The listing builds one solid part. Answer for the finished solid, in the listing's coordinates (mm). A direction names the side the tool comes from. Give positions to 0.01 mm unless a question says otherwise; leave off trailing zeros. Order: outer loops, then holes, each group sorted by start corner. A loop starts at its lowest first (then second) coordinate and runs counter-clockwise, first axis right, second up.
```python
from build123d import *

# Parameters (mm, degrees)
ESQUISSE1_W              = 150
ESQUISSE1_H              = 240
BOSS_EXTRU_1_DEPTH       = 50
ENL_V_MAT_EXTRU_1_DEPTH  = 42
ESQUISSE3_W              = 101
ESQUISSE3_H              = 165.5
ENL_V_MAT_EXTRU_2_DEPTH  = 151.083310198
CONG_1_R                 = 5
ESQUISSE4_R              = 2.8
ENL_V_MAT_EXTRU_3_DEPTH  = 15
ENL_V_MAT_EXTRU_4_DEPTH  = 199.494332413
ESQUISSE7_R              = 2.3
ENL_V_MAT_EXTRU_5_DEPTH  = 5
ESQUISSE6_R              = 2
ENL_V_MAT_EXTRU_6_DEPTH  = 5
ESQUISSE8_W              = 5
ESQUISSE8_H              = 40
ENL_V_MAT_EXTRU_7_DEPTH  = 7
ESQUISSE9_R              = 4
BOSS_EXTRU_2_DEPTH       = 9
ESQUISSE10_R             = 2.3
ENL_V_MAT_EXTRU_8_DEPTH  = 8
ESQUISSE11_W             = 101
ESQUISSE11_H             = 11
ENL_V_MAT_EXTRU_9_DEPTH  = 3
BOSS_EXTRU_3_START       = 10
ESQUISSE13_R             = 4
ESQUISSE13_R_2           = 2.3
ESQUISSE13_R_3           = 2
BOSS_EXTRU_3_DEPTH       = 10
ESQUISSE14_R             = 2.3
ENL_V_MAT_EXTRU_10_DEPTH = 6.7


with BuildPart() as part:
    # Esquisse1 → Boss.-Extru.1 (new body)
    with BuildSketch(Plane.XY):
        Rectangle(ESQUISSE1_W, ESQUISSE1_H)
    extrude(amount=BOSS_EXTRU_1_DEPTH)

    # Esquisse2 → Enl_v. mat.-Extru.1 (cut)
    with BuildSketch(Plane(origin=(0, 0, 0), x_dir=(-1, 0, 0), z_dir=(0, 0, -1))):
        with BuildLine():
            Line((-70, -110), (-70, 110))
            Line((-70, 110), (-67, 110))
            ThreePointArc((-67, 110), (-65.585786438, 110.585786438), (-65, 112))
            Line((-65, 112), (-65, 115))
            Line((-65, 115), (65, 115))
            Line((65, 115), (65, 112))
            ThreePointArc((65, 112), (65.585786438, 110.585786438), (67, 110))
            Line((67, 110), (70, 110))
            Line((70, 110), (70, -110))
            Line((70, -110), (26, -110))
            ThreePointArc((26, -110), (25.292893219, -110.292893219), (25, -111))
            Line((25, -111), (25, -115))
            Line((25, -115), (-65, -115))
            Line((-65, -115), (-65, -112))
            ThreePointArc((-65, -112), (-65.585786438, -110.585786438), (-67, -110))
            Line((-67, -110), (-70, -110))
        make_face()
    extrude(amount=-ENL_V_MAT_EXTRU_1_DEPTH, mode=Mode.SUBTRACT)

    # Esquisse3 → Enl_v. mat.-Extru.2 (cut, through all)
    with BuildSketch(Plane.XY.offset(50)):
        with Locations((0, 27.25)):
            Rectangle(ESQUISSE3_W, ESQUISSE3_H)
    extrude(amount=-ENL_V_MAT_EXTRU_2_DEPTH, mode=Mode.SUBTRACT)

    # Cong_1
    cong_1_edges = [part.edges().sort_by_distance(p)[0] for p in [
        (-75, 120, 25),
        (75, 120, 25),
        (75, -120, 25),
        (-75, -120, 25),
    ]]
    fillet(cong_1_edges, radius=CONG_1_R)

    # Esquisse4 → Enl_v. mat.-Extru.3 (cut)
    with BuildSketch(Plane(origin=(0, 0, 0), x_dir=(-1, 0, 0), z_dir=(0, 0, -1))):
        with Locations((-70, 115)):
            Circle(ESQUISSE4_R)
        with Locations((70, 115)):
            Circle(ESQUISSE4_R)
        with Locations((70, -115)):
            Circle(ESQUISSE4_R)
        with Locations((-70, -115)):
            Circle(ESQUISSE4_R)
    extrude(amount=-ENL_V_MAT_EXTRU_3_DEPTH, mode=Mode.SUBTRACT)

    # Esquisse5 → Enl_v. mat.-Extru.4 (cut, through all)
    with BuildSketch(Plane(origin=(75, 0, 0), x_dir=(0, 0, -1), z_dir=(1, 0, 0))):
        with BuildLine():
            Line((-37, 55), (-18.584929033, 78.683014193))
            ThreePointArc((-18.584929033, 78.683014193), (-14.375120517, 79.209808516), (-13.848326194, 75))
            Line((-13.848326194, 75), (-32.263397161, 51.316985807))
            ThreePointArc((-32.263397161, 51.316985807), (-36.473205677, 50.790191484), (-37, 55))
        make_face()
        with BuildLine():
            Line((-37, 5), (-18.584929033, 28.683014193))
            ThreePointArc((-18.584929033, 28.683014193), (-14.375120517, 29.209808516), (-13.848326194, 25))
            Line((-13.848326194, 25), (-32.263397161, 1.316985807))
            ThreePointArc((-32.263397161, 1.316985807), (-36.473205677, 0.790191484), (-37, 5))
        make_face()
        with BuildLine():
            Line((-37, -45), (-18.584929033, -21.316985807))
            ThreePointArc((-18.584929033, -21.316985807), (-14.375120517, -20.790191484), (-13.848326194, -25))
            Line((-13.848326194, -25), (-32.263397161, -48.683014193))
            ThreePointArc((-32.263397161, -48.683014193), (-36.473205677, -49.209808516), (-37, -45))
        make_face()
    extrude(amount=-ENL_V_MAT_EXTRU_4_DEPTH, mode=Mode.SUBTRACT)

    # Esquisse7 → Enl_v. mat.-Extru.5 (cut)
    with BuildSketch(Plane(origin=(0, 0, 42), x_dir=(-1, 0, 0), z_dir=(0, 0, -1))):
        with Locations((-57, 105.8)):
            Circle(ESQUISSE7_R)
        with Locations((-57, -51.3)):
            Circle(ESQUISSE7_R)
        with Locations((57, 105.8)):
            Circle(ESQUISSE7_R)
        with Locations((57, -51.3)):
            Circle(ESQUISSE7_R)
    extrude(amount=-ENL_V_MAT_EXTRU_5_DEPTH, mode=Mode.SUBTRACT)

    # Esquisse6 → Enl_v. mat.-Extru.6 (cut)
    with BuildSketch(Plane(origin=(0, 0, 42), x_dir=(-1, 0, 0), z_dir=(0, 0, -1))):
        with Locations((-14.8, -79.815913119)):
            Circle(ESQUISSE6_R)
        with Locations((13, -105.015913119)):
            Circle(ESQUISSE6_R)
    extrude(amount=-ENL_V_MAT_EXTRU_6_DEPTH, mode=Mode.SUBTRACT)

    # Esquisse8 → Enl_v. mat.-Extru.7 (cut)
    with BuildSketch(Plane(origin=(0, 0, 42), x_dir=(-1, 0, 0), z_dir=(0, 0, -1))):
        with Locations((53, -27.5)):
            Rectangle(ESQUISSE8_W, ESQUISSE8_H)
    extrude(amount=-ENL_V_MAT_EXTRU_7_DEPTH, mode=Mode.SUBTRACT)

    # Esquisse9 → Boss.-Extru.2 (add)
    with BuildSketch(Plane(origin=(0, 0, 42), x_dir=(-1, 0, 0), z_dir=(0, 0, -1))):
        with Locations((-60, 97)):
            Circle(ESQUISSE9_R)
        with Locations((60, 97)):
            Circle(ESQUISSE9_R)
        with Locations((60, -33)):
            Circle(ESQUISSE9_R)
        with Locations((-60, -33)):
            Circle(ESQUISSE9_R)
    extrude(amount=BOSS_EXTRU_2_DEPTH)

    # Esquisse10 → Enl_v. mat.-Extru.8 (cut)
    with BuildSketch(Plane(origin=(0, 0, 33), x_dir=(-1, 0, 0), z_dir=(0, 0, -1))):
        with Locations((-60, 97)):
            Circle(ESQUISSE10_R)
        with Locations((60, 97)):
            Circle(ESQUISSE10_R)
        with Locations((60, -33)):
            Circle(ESQUISSE10_R)
        with Locations((-60, -33)):
            Circle(ESQUISSE10_R)
    extrude(amount=-ENL_V_MAT_EXTRU_8_DEPTH, mode=Mode.SUBTRACT)

    # Esquisse11 → Enl_v. mat.-Extru.9 (cut)
    with BuildSketch(Plane(origin=(0, 0, 42), x_dir=(-1, 0, 0), z_dir=(0, 0, -1))):
        with Locations((0, -61)):
            Rectangle(ESQUISSE11_W, ESQUISSE11_H)
    extrude(amount=-ENL_V_MAT_EXTRU_9_DEPTH, mode=Mode.SUBTRACT)

    # Esquisse13 → Boss.-Extru.3 (add)
    # profile 1 of 2: a face of its own
    with BuildSketch(Plane(origin=(0, 0, 42), x_dir=(-1, 0, 0), z_dir=(0, 0, -1)).offset(BOSS_EXTRU_3_START)):
        with Locations((-14.8, -79.815913119)):
            Circle(ESQUISSE13_R)
        with Locations((-14.8, -79.815913119)):
            Circle(ESQUISSE13_R_2, mode=Mode.SUBTRACT)
    # profile 2 of 2: a face of its own
    with BuildSketch(Plane(origin=(0, 0, 42), x_dir=(-1, 0, 0), z_dir=(0, 0, -1)).offset(BOSS_EXTRU_3_START)):
        with Locations((13, -105.015913119)):
            Circle(ESQUISSE13_R)
        with Locations((13, -105.015913119)):
            Circle(ESQUISSE13_R_3, mode=Mode.SUBTRACT)
    extrude(amount=-BOSS_EXTRU_3_DEPTH)

    # Esquisse14 → Enl_v. mat.-Extru.10 (cut)
    with BuildSketch(Plane(origin=(0, -110, 0), x_dir=(1, 0, 0), z_dir=(0, 1, 0))):
        with Locations(Location((-63.627600244, -37.7, 0), (0, 0, 180))):
            Circle(ESQUISSE14_R)
        with Locations(Location((-63.627600244, -4.8, 0), (0, 0, 180))):
            Circle(ESQUISSE14_R)
        with Locations(Location((-20.327600244, -4.8, 0), (0, 0, 180))):
            Circle(ESQUISSE14_R)
    extrude(amount=-ENL_V_MAT_EXTRU_10_DEPTH, mode=Mode.SUBTRACT)


solid = part.part
```
1) Straight lines are drawn through the part: probe 1 along Y at (x, z) = (57, 45.3); probe 2 along Y at (x, z) = (-17, 30.5); probe 3 along Y at (x, z) = (56.5, 46.5) (3 decimals). For each, find the intervals that lie inside material, in ascending order.
Geometry says:
probe 1: y = -120 to -53.6, -49 to 103.5, 108.1 to 120
probe 2: y = -120 to -115, 115 to 120
probe 3: y = -120 to -53.545, -49.055 to 103.555, 108.045 to 120
2) Find section A-A (y = 46). Write down the section's boundary in (x, z), then the cut area to 3 significant figures.
Geometry says:
outline: (-75, 0) - (-70, 0) - (-70, 42) - (-50.5, 42) - (-50.5, 50) - (-75, 50) - close; (50.5, 42) - (70, 42) - (70, 0) - (75, 0) - (75, 50) - (50.5, 50) - close
area: 812 mm2
3) For a pull along Y with two mould halves and no side action, classify faces 4 (the cylindrical face through (-74, 118, 25)), 5 (the flat face through (72.5, -33.3, 27.9)) as +Y half, -Y half, draft (parallel to the pull), parting line (faces both ways), or undercut.
Geometry says:
face 4: +Y half
face 5: undercut
4) Find section B-B (x = -40). Write down the section's boundary in (y, z), then the cut area to 3 significant figures.
Geometry says:
outline: (-120, 0) - (-110, 0) - (-110, 42) - (-66.5, 42) - (-66.5, 45) - (-55.5, 45) - (-55.5, 50) - (-120, 50) - close; (110, 42) - (115, 42) - (115, 0) - (120, 0) - (120, 50) - (110, 50) - close
area: 1,190 mm2
5) Given P1, Ø9, axis at x = 61.5, y = 95, coming from the -Z side; P2, Ø1.2, axis at x = -13.5, y = -105, coming from the -Z side; P3, Ø2.5, axis at x = 13.5, y = -78.5, coming from the -Z side, each flat-ended and moving along its own axis, determine where each tip first touches the part or whether it passes through.
Geometry says:
P1: stops at z = 33
P2: stops at z = 47
P3: stops at z = 32
6) A tool of negligible diameter and unlimited length cuts with its end or side. For faces 1 (the cylindrical face through (72.54, -49.25, 36.42)), 2 (the cylindrical face through (-61.93, -113.3, 39.25)), 3 (the flat face through (70, 115, 15)), from which of +Z, -Z, +X, -X, +Y, -Y can it reach the whole face along a straight path? Write none if from no direction.
Geometry says:
face 1: +X, -X
face 2: none
face 3: -Z
